The listing builds one solid part. Answer for the finished solid, in the listing's coordinates (mm). Face numbers are marked on the shaded views. Coordinates: 2 decimals unless noted, no trailing zeros. Order: outer loops, then holes, each group sorted by start corner. A loop starts at its lowest first (then second) coordinate and runs counter-clockwise, first axis right, second up. Notation, with made-up numbers: (-5, 7) -> (1, 7) arc R22 ccw to (1, 21) -> close; hole circle Ø1 at (80, 40.5). An arc over 180 degrees is marked (long way). Write item = value, one per line.
from build123d import *

# Parameters (mm, degrees)
F0_R      = 20.140817
F1_DEPTH  = 50
F2_R      = 15.312495
F3_DEPTH  = 49
F1_FACE_R = 20.140817
F4_DEPTH  = 25


with BuildPart() as f1:
    # F0 (on Top) → F1 (new body)
    with BuildSketch(Plane.XY):
        Circle(F0_R)
    extrude(amount=F1_DEPTH)

    # F2 (on Top) → F3 (cut)
    with BuildSketch(Plane.XY):
        Circle(F2_R)
    extrude(amount=F3_DEPTH, mode=Mode.SUBTRACT)

    # F1_face (on face) → F4 (join)
    with BuildSketch(Plane.XY.offset(50)):
        Circle(F1_FACE_R)
    extrude(amount=F4_DEPTH)


solid = f1.part
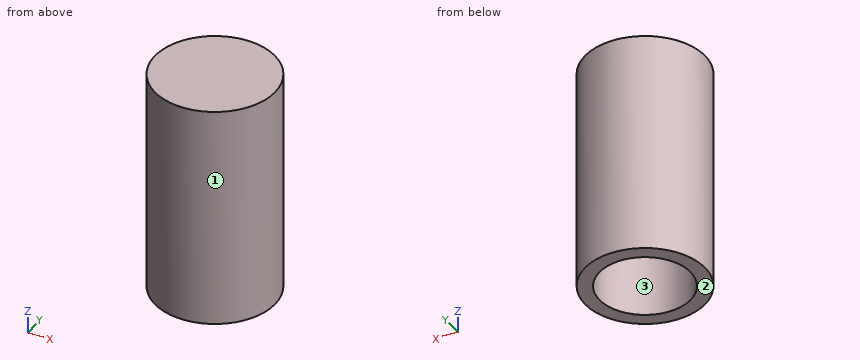
Q1. Each of these flat-tipped pins is pushed along its axis until it touches: pin 1 Ø1.5 at (x, z) = (-1.5, 32.5) entering from +Y; pin 2 Ø4 at (x, z) = (15, 54.5) entering from +Y; pin 3 Ø8 at (y, z) = (-0.5, 17) entering from -X; pin 4 Ø10 at (y, z) = (7, 49.5) entering from -X. Where does it stop, or does it pass through?
The answers:
pin_1 = 20.13
pin_2 = 15.38
pin_3 = -20.14
pin_4 = -20.04
Q2. Section C-C, the plane x = -12.5 is taken. Give the vertices of the cut face in (y, z), plus the area to 3 significant figures.
The answers:
outline = (-15.79, 0) -> (-8.84, 0) -> (-8.84, 49) -> (8.84, 49) -> (8.84, 0) -> (15.79, 0) -> (15.79, 75) -> (-15.79, 75) -> close
area = 1,500 mm2
Q3. Section D-D, the plane x = 18.5 is taken. Give the vertices of the cut face in (y, z), plus the area to 3 significant figures.
The answers:
outline = (-7.96, 0) -> (7.96, 0) -> (7.96, 75) -> (-7.96, 75) -> close
area = 1,190 mm2
Q4. Find the intervals of material crossed by line 1 along Y through (x, z) = (0, 19); line 2 along Z through (x, y) = (-1, -11); line 3 along X through (y, z) = (8.5, 17), in increasing order.
The answers:
line_1 = -20.14 to -15.31, 15.31 to 20.14
line_2 = 49 to 75
line_3 = -18.26 to -12.74, 12.74 to 18.26
Q5. The mould has two halves that part along X. Classify the marked faces 1, 2 and 3: released by +X, released by -X, zero draft, split by the parting line, or undercut.
The answers:
face_1 = split by the parting line
face_2 = zero draft
face_3 = undercut
Q6. Section A-A, the plane y = 0 is taken. Give the vertices of the cut face in (x, z), plus the area to 3 significant figures.
The answers:
outline = (-20.14, 0) -> (-15.31, 0) -> (-15.31, 49) -> (15.31, 49) -> (15.31, 0) -> (20.14, 0) -> (20.14, 75) -> (-20.14, 75) -> close
area = 1,520 mm2
Q7. Section B-B, the plane z = 19 is taken. Give the vertices of the cut face in (x, y) (1 decimal).
The answers:
outline = circle Ø40.3 at (0, 0); hole circle Ø30.6 at (0, 0)
